The model under review builds one solid part; all positions refer to its coordinate system, in mm. Coordinates: 2 decimals unless noted, no trailing zeros. Order: outer loops, then holes, each group sorted by start corner. A loop starts at its lowest first (then second) coordinate and runs counter-clockwise, first axis right, second up. Notation, with made-up numbers: M -29,-26 L 17,-26 A11 ccw 17,-16 Z; hole C -33.75,-1.75 d10. An arc over 180 degrees is marked long. Answer as CSV lines item,"result". Start each with the question number.
Q1. Consider section B-B on z = 9. Write out the cut boundary in (x, y), and give its area (3 significant figures).
Q2. For P1, Ø5, axis at x = -177.38, z = 32.89, coming from the -Y side; P2, Ø2.5, axis at x = -254.88, y = 3.5, coming from the +Z side; P3, Ø2, axis at x = -166, z = 23.5, coming from the +Y side; P4, Ø2, axis at y = 4, z = 6, coming from the -X side, all flat-tipped, find the tip position at first contact; note any pin that passes through.
Q3. Consider section C-C on x = -189. Write out the cut boundary in (y, z).
Q4. Consider section A-A on y = 14.5. Write out the cut boundary in (x, z), and give its area (3 significant figures).
Q5. Consider section D-D on x = -119.5. Write out the cut boundary in (y, z).
Q6. Wall thickness on L1, parallel to Z at x = -175, y = 4.25; L2, parallel to X at y = 20, z = -22.5; L3, parallel to X at y = 3.5, z = 25: over which ranges is each line inside the solid? List them lowest first. Write a range as [from, to].
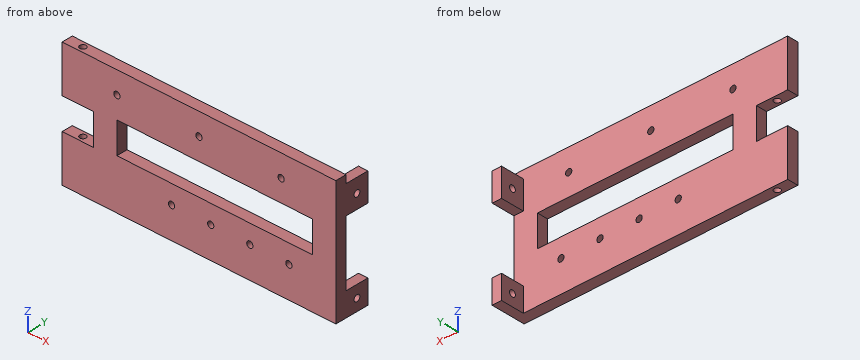
from build123d import *

# Parameters (mm, degrees)
SKETCH1_W               = 175
SKETCH1_H               = 80
BOSS_EXTRUDE1_DEPTH     = 7
SKETCH2_R               = 2
CUT_EXTRUDE1_DEPTH      = 10
SKETCH3_W               = 125
SKETCH3_H               = 20
CUT_EXTRUDE2_DEPTH      = 1
SKETCH7_W               = 6
SKETCH7_H               = 15.226692755
SKETCH7_H_2             = 18
BOSS_EXTRUDE3_DEPTH     = 15
SKETCH8_R               = 2
CUT_EXTRUDE4_DEPTH      = 15
SKETCH9_W               = 20
SKETCH9_H               = 20
CUT_EXTRUDE5_DEPTH      = 15
SKETCH10_R              = 2
CUT_EXTRUDE7_DEPTH      = 51
CUT_EXTRUDE7_DEPTH_BACK = 31
SKETCH3_3_W             = 125
SKETCH3_3_H             = 20
CUT_EXTRUDE8_DEPTH      = 10
SKETCH11_R              = 2
CUT_EXTRUDE9_DEPTH      = 10


with BuildPart() as part:
    # Sketch1 → Boss-Extrude1 (new body)
    with BuildSketch(Plane(origin=(0, 0, 0), x_dir=(1, 0, 0), z_dir=(0, 1, 0))):
        with Locations((-2.383449883, -6.993006993)):
            Rectangle(SKETCH1_W, SKETCH1_H)
    extrude(amount=BOSS_EXTRUDE1_DEPTH)

    # Sketch2 → Cut-Extrude1 (cut)
    with BuildSketch(Plane(origin=(0, 7, 0), x_dir=(1, 0, 0), z_dir=(0, 1, 0))):
        with Locations((-54.883449883, -32.893006993)):
            Circle(SKETCH2_R)
        with Locations((-2.383449883, -32.893006993)):
            Circle(SKETCH2_R)
        with Locations((50.116550117, -32.893006993)):
            Circle(SKETCH2_R)
    extrude(amount=-CUT_EXTRUDE1_DEPTH, mode=Mode.SUBTRACT)

    # Sketch3 → Cut-Extrude2 (cut)
    with BuildSketch(Plane(origin=(0, 7, 0), x_dir=(1, 0, 0), z_dir=(0, 1, 0))):
        with Locations((-12.383449883, -8.993006993)):
            Rectangle(SKETCH3_W, SKETCH3_H)
    extrude(amount=-CUT_EXTRUDE2_DEPTH, mode=Mode.SUBTRACT)

    # Sketch7 → Boss-Extrude3 (add)
    with BuildSketch(Plane(origin=(0, 7, 0), x_dir=(1, 0, 0), z_dir=(0, 1, 0))):
        with Locations((-86.883449883, 25.39364663)):
            Rectangle(SKETCH7_W, SKETCH7_H)
        with Locations((-86.883449883, -32.993006993)):
            Rectangle(SKETCH7_W, SKETCH7_H_2)
    extrude(amount=BOSS_EXTRUDE3_DEPTH)

    # Sketch8 → Cut-Extrude4 (cut)
    with BuildSketch(Plane(origin=(-83.883449883, 0, 0), x_dir=(0, 0, -1), z_dir=(1, 0, 0))):
        with Locations((25.506993007, 14.5)):
            Circle(SKETCH8_R)
        with Locations((-32.993006993, 14.5)):
            Circle(SKETCH8_R)
    extrude(amount=-CUT_EXTRUDE4_DEPTH, mode=Mode.SUBTRACT)

    # Sketch9 → Cut-Extrude5 (cut)
    with BuildSketch(Plane.XZ):
        with Locations((75.116550117, 6.993006993)):
            Rectangle(SKETCH9_W, SKETCH9_H)
    extrude(amount=-CUT_EXTRUDE5_DEPTH, mode=Mode.SUBTRACT)

    # Sketch10 → Cut-Extrude7 (cut, two sides)
    with BuildSketch(Plane.XY.offset(-3.006993007)) as cut_extrude7_sk:
        with Locations((75.116550117, 3.5)):
            Circle(SKETCH10_R)
    extrude(amount=CUT_EXTRUDE7_DEPTH, mode=Mode.SUBTRACT)
    extrude(cut_extrude7_sk.sketch, amount=-CUT_EXTRUDE7_DEPTH_BACK, mode=Mode.SUBTRACT)

    # Sketch3<3> → Cut-Extrude8 (cut)
    with BuildSketch(Plane(origin=(0, 7, 0), x_dir=(1, 0, 0), z_dir=(0, 1, 0))):
        with Locations((-12.383449883, -8.993006993)):
            Rectangle(SKETCH3_3_W, SKETCH3_3_H)
    extrude(amount=-CUT_EXTRUDE8_DEPTH, mode=Mode.SUBTRACT)

    # Sketch11 → Cut-Extrude9 (cut)
    with BuildSketch(Plane(origin=(0, 7, 0), x_dir=(1, 0, 0), z_dir=(0, 1, 0))):
        with Locations((-59.883449883, 13.006993007)):
            Circle(SKETCH11_R)
        with Locations((-34.883449883, 13.006993007)):
            Circle(SKETCH11_R)
        with Locations((-9.883449883, 13.006993007)):
            Circle(SKETCH11_R)
        with Locations((15.116550117, 13.006993007)):
            Circle(SKETCH11_R)
    extrude(amount=-CUT_EXTRUDE9_DEPTH, mode=Mode.SUBTRACT)


with BuildPart() as body_2:
    # Mirror2: mirrored copy
    add(part.part.mirror(Plane(origin=(-89.883449883, 7, -33.006993007), x_dir=(0, 0, 1), z_dir=(1, 0, 0))))


solid = body_2.part
Evaluation:
1,outline,"M -244.88,0 L -229.88,0 L -229.88,7 L -244.88,7 Z; M -104.88,0 L -89.88,0 L -89.88,7 L -104.88,7 Z"
1,area,"210 mm²"
2,P1,"stops at y = 0"
2,P2,"passes through"
2,P3,"stops at y = 7"
2,P4,"stops at x = -244.88"
3,outline,"M 0,-33.01 L 7,-33.01 L 7,-1.01 L 0,-1.01 Z; M 0,18.99 L 7,18.99 L 7,46.99 L 0,46.99 Z"
4,outline,"M -95.88,-33.01 L -89.88,-33.01 L -89.88,-27.51 L -95.88,-27.51 Z; M -95.88,-23.51 L -89.88,-23.51 L -89.88,-17.78 L -95.88,-17.78 Z; M -95.88,23.99 L -89.88,23.99 L -89.88,30.99 L -95.88,30.99 Z; M -95.88,34.99 L -89.88,34.99 L -89.88,41.99 L -95.88,41.99 Z"
4,area,"151 mm²"
5,outline,"M 0,-33.01 L 7,-33.01 L 7,-14.97 L 0,-14.97 Z; M 0,-11.04 L 7,-11.04 L 7,-1.01 L 0,-1.01 Z; M 0,18.99 L 7,18.99 L 7,46.99 L 0,46.99 Z"
6,L1,"z = [-33.01, -1.01], [18.99, 46.99]"
6,L2,"x = [-95.88, -89.88]"
6,L3,"x = [-264.88, -256.88], [-252.88, -89.88]"
